```python
from build123d import *

# Parameters (mm, degrees)
SKETCH_R     = 30
PAD_DEPTH    = 5
SKETCH001_R  = 10
PAD001_DEPTH = 4
SKETCH002_R  = 2.25
POCKET_DEPTH = 9
FILLET_R     = 2.5


with BuildPart() as part:
    # Sketch → Pad (new body)
    with BuildSketch(Plane.XY):
        Circle(SKETCH_R)
    extrude(amount=PAD_DEPTH)

    # Sketch001 (on Face3 of Pad) → Pad001 (join)
    with BuildSketch(Plane.XY.offset(5)):
        Circle(SKETCH001_R)
    extrude(amount=PAD001_DEPTH)

    # Sketch002 (on Face5 of Pad001) → Pocket (cut)
    with BuildSketch(Plane.XY.offset(9)):
        Circle(SKETCH002_R)
    extrude(amount=-POCKET_DEPTH, mode=Mode.SUBTRACT)

    # Fillet
    fillet_edges = [part.edges().sort_by_distance(p)[0] for p in [
        (-10, 0, 5),
    ]]
    fillet(fillet_edges, radius=FILLET_R)


solid = part.part
```
Geometry: final body of the model. Coordinates: model frame, mm. A direction names the side the tool comes from. Coordinates: 2 decimals unless noted, no trailing zeros. Order: outer loops, then holes, each group sorted by start corner. A loop starts at its lowest first (then second) coordinate and runs counter-clockwise, first axis right, second up. Notation, with made-up numbers: (11.25, 29.25) -> (35.25, 29.25) arc R15 cw to (35.25, 35.25) -> close; hole circle Ø9 at (-25, -18.75). An arc over 180 degrees is marked (long way). Write item = value, one per line.
(1) Access query for faces 4 (the cylindrical face through (-2.17, -9.76, 8.24)), 5 (the flat face through (6, 0, 0)). Directions: +Z, -Z, +X, -X, +Y, -Y. A direction counts if a zero-diameter tool reaches every point of the face in a straight line with its end or side. Return the directions, or none.
Solved:
face_4 = +Z
face_5 = -Z, +X, -X, +Y, -Y
(2) Line query: line 1 (Y direction, x = 0, z = 3.25); line 2 (Z direction, x = 3, y = -26); line 3 (Y direction, x = 0, z = 5.75). Output: solid intervals per line, ascending.
Solved:
line_1 = -30 to -2.25, 2.25 to 30
line_2 = 0 to 5
line_3 = -10.71 to -2.25, 2.25 to 10.71
(3) Pull-direction query (X, two-part tool) for faces 1 (the flat face through (13, 0, 5)), 2 (the cylindrical face through (-0.29, 2.23, 4.56)), 3 (the cylindrical face through (-29.97, 1.32, 2.46)); classes: pulls with the +X half, pulls with the -X half, needs draft (parallel to the pull), parting line crosses it, or undercut.
Solved:
face_1 = needs draft
face_2 = undercut
face_3 = parting line crosses it
(4) Pin query (flat end, axial travel): pin 1 Ø5 at (x, z) = (7.5, 3) entering from -Y; pin 2 Ø2 at (y, z) = (7, 4) entering from +X; pin 3 Ø1 at (x, z) = (-4.5, 8) entering from +Y. Return the tip coordinate at first contact, or that it passes through.
Solved:
pin_1 = -29.58
pin_2 = 29.39
pin_3 = 9.17
(5) Cut plane C-C on x = -18. Return loops of the section in (y, z), plus the area to 3 significant figures.
Solved:
outline = (-24, 0) -> (24, 0) -> (24, 5) -> (-24, 5) -> close
area = 240 mm²
(6) Cut plane D-D on x = 21.5. Return loops of the section in (y, z), plus the area to 3 significant figures.
Solved:
outline = (-20.92, 0) -> (20.92, 0) -> (20.92, 5) -> (-20.92, 5) -> close
area = 209 mm²
(7) Cut plane A-A on y = 0. Return loops of the section in (x, z), plus the area to 3 significant figures.
Solved:
outline = (-30, 0) -> (-2.25, 0) -> (-2.25, 9) -> (-10, 9) -> (-10, 7.5) arc R2.5 cw to (-12.5, 5) -> (-30, 5) -> close; (2.25, 0) -> (30, 0) -> (30, 5) -> (12.5, 5) arc R2.5 cw to (10, 7.5) -> (10, 9) -> (2.25, 9) -> close
area = 342 mm²
